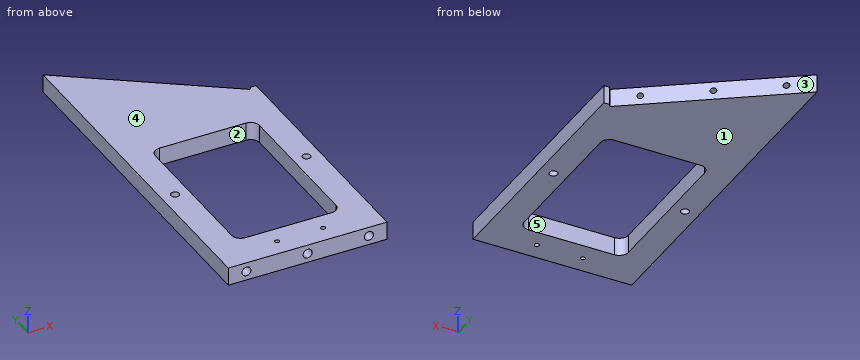
from build123d import *

# Parameters (mm, degrees)
EXTRUDE_1_DEPTH        = 10
PATTERN_LINEAR_1_COUNT = 3
PATTERN_LINEAR_1_PITCH = 36
CUT_EXTRUDE_1_DEPTH    = 160.432744146
PATTERN_LINEAR_2_COUNT = 3
PATTERN_LINEAR_2_PITCH = 33.8
SKETCH_7_R             = 2.25
CUT_EXTRUDE_2_DEPTH    = 160.432744146
HOLE_WIZARD_M3_1_D     = 2.5
PATTERN_LINEAR_3_COUNT = 2
PATTERN_LINEAR_3_PITCH = 25.4


with BuildPart() as part:
    # 草图1 → 凸台-拉伸1 (new body)
    with BuildSketch(Plane.XY):
        Polygon((0, 0), (-83.451271177, 58.650535708), (-83.451271177, -135.479464292), (4.150010504, -135.479464292), (4.150010504, 1.636299435), (1.150010504, 1.636299435), align=None)
    extrude(amount=EXTRUDE_1_DEPTH)

    # 草图2 → M4 螺纹孔1 (revolve, cut)
    with BuildSketch(Plane(origin=(-12.272245761, 8.625078781, 5), x_dir=(-0.8181497174250271, 0.5750052520432736, 0), z_dir=(0, 0, 1))):
        Polygon((0, 0), (0, 11.091420021), (1.65, 10.1), (1.65, 0), align=None)
    hole_wizard_m4_1 = revolve(axis=Axis((-8.620962411, 13.820329486, 5), (-0.5750052520432737, -0.818149717425027, 0)), mode=Mode.SUBTRACT)

    # 阵列(线性)1: M4 螺纹孔1 ×3
    with Locations(*[Vector(-0.8181497174250268, 0.5750052520432738, 0) * (i * PATTERN_LINEAR_1_PITCH) for i in range(1, PATTERN_LINEAR_1_COUNT)]):
        add(hole_wizard_m4_1, mode=Mode.SUBTRACT)

    # 草图4 → 切除-拉伸1 (cut, through all)
    with BuildSketch(Plane.XY.offset(10)):
        with BuildLine():
            Line((-63.451271177, -115.479464292), (-15.849989496, -115.479464292))
            ThreePointArc((-15.849989496, -115.479464292), (-12.31445559, -114.014998198), (-10.849989496, -110.479464292))
            Line((-10.849989496, -110.479464292), (-10.849989496, -30.479464292))
            ThreePointArc((-10.849989496, -30.479464292), (-12.31445559, -26.943930386), (-15.849989496, -25.479464292))
            Line((-15.849989496, -25.479464292), (-63.451271177, -25.479464292))
            ThreePointArc((-63.451271177, -25.479464292), (-66.986805083, -26.943930386), (-68.451271177, -30.479464292))
            Line((-68.451271177, -30.479464292), (-68.451271177, -110.479464292))
            ThreePointArc((-68.451271177, -110.479464292), (-66.986805083, -114.014998198), (-63.451271177, -115.479464292))
        make_face()
    extrude(amount=-CUT_EXTRUDE_1_DEPTH, mode=Mode.SUBTRACT)

    # 草图5 → M6 螺纹孔1 (revolve, cut)
    with BuildSketch(Plane(origin=(-5.849989496, -135.479464292, 5), x_dir=(0, 0, -1), z_dir=(1, 0, 0))):
        Polygon((0, 0), (0, 16.502151548), (2.5, 15), (2.5, 0), align=None)
    hole_wizard_m6_1 = revolve(axis=Axis((-5.849989496, -141.829464292, 5), (0, 1, 0)), mode=Mode.SUBTRACT)

    # 阵列(线性)2: M6 螺纹孔1 ×3
    with Locations(*[(-i * PATTERN_LINEAR_2_PITCH, 0, 0) for i in range(1, PATTERN_LINEAR_2_COUNT)]):
        add(hole_wizard_m6_1, mode=Mode.SUBTRACT)

    # 草图7 → 切除-拉伸2 (cut, through all)
    with BuildSketch(Plane.XY.offset(10)):
        with Locations((-75.951271177, -65.479464292)):
            Circle(SKETCH_7_R)
        with Locations((-3.349989496, -65.479464292)):
            Circle(SKETCH_7_R)
    extrude(amount=-CUT_EXTRUDE_2_DEPTH, mode=Mode.SUBTRACT)

    # M3 螺纹孔1 (through all)
    with Locations(Plane(origin=(0, 0, 0), x_dir=(-1, 0, 0), z_dir=(0, 0, -1))):
        with Locations((25.849989496, -125.479464292)):
            hole_wizard_m3_1 = Hole(HOLE_WIZARD_M3_1_D / 2)

    # 阵列(线性)3: M3 螺纹孔1 ×2
    with Locations(*[(-i * PATTERN_LINEAR_3_PITCH, 0, 0) for i in range(1, PATTERN_LINEAR_3_COUNT)]):
        add(hole_wizard_m3_1, mode=Mode.SUBTRACT)


solid = part.part
The model under review builds one solid part; all positions refer to its coordinate system, in mm. Face numbers are marked on the shaded views. A direction names the side the tool comes from. Round coordinates to 2 decimals unless told otherwise and drop trailing zeros. Loops run counter-clockwise (first coordinate to the right, second up) from the corner with the lowest first, then second, coordinate; pieces in that order, holes last. Notation, with made-up numbers: (39.25, -11.5) -> (96.25, -11.5) arc R22 cw to (96.25, 24.5) -> close; hole circle Ø4 at (89.25, 72). An arc over 180 degrees is marked (long way). One line per question, with ' | ' between items. Start each with the question number.
Item 1: Machinability: for the marked faces 1 and 2, which of the approach directions +Z, -Z, +X, -X, +Y, -Y give a long, thin tool a straight path to every point of the face, cutting with its end or side? Answer none if there is none.
Item 2: For pin 1 (6 mm diameter, centred on x = -72, z = 5.5, fed in from +Y); pin 2 (2 mm diameter, centred on x = -51.25, y = -125.48, fed in from +Z); pin 3 (4 mm diameter, centred on x = -73.45, z = 5, fed in from +Y); pin 4 (7 mm diameter, centred on x = -3.35, y = -65.48, fed in from +Z), all flat-tipped, find the tip position at first contact; note any pin that passes through.
Item 3: Add section B-B, the plane x = -32. Write out the cut boundary in (y, z).
Item 4: Draft analysis for pull direction Y (two halves, no side actions). For the marked faces 3, 4 and 5, state which applies: +Y half, -Y half, draft (parallel to the pull), parting line (faces both ways), or undercut.
Item 5: Add section A-A, the plane y = -42. Write out the cut boundary in (x, z), then the cut area to 3 significant figures.
Item 6: Wall thickness on line 1 along X through (y, z) = (-127.5, 5); line 2 along X through (y, z) = (-78, 2.25); line 3 along X through (y, z) = (-64, 5): over which ranges is each line inside the solid? List them lowest first. Write a range as [from, to].
Return value:
1) face 1: -Z, +X, -X, +Y, -Y | face 2: +Z, -Z
2) pin 1: stops at y = 52.71 | pin 2: passes through | pin 3: stops at y = 53.03 | pin 4: stops at z = 10
3) outline: (-135.48, 0) -> (-115.48, 0) -> (-115.48, 10) -> (-135.48, 10) -> close; (-25.48, 0) -> (22.49, 0) -> (22.49, 10) -> (-25.48, 10) -> close
4) face 3: +Y half | face 4: draft | face 5: undercut
5) outline: (-83.45, 0) -> (-68.45, 0) -> (-68.45, 10) -> (-83.45, 10) -> close; (-10.85, 0) -> (4.15, 0) -> (4.15, 10) -> (-10.85, 10) -> close | area: 300 mm2
6) line 1: x = [-83.45, -75.95], [-70.95, -42.15], [-37.15, -8.35], [-3.35, 4.15] | line 2: x = [-83.45, -68.45], [-10.85, 4.15] | line 3: x = [-83.45, -77.65], [-74.26, -68.45], [-10.85, -5.05], [-1.65, 4.15]
